```python
from build123d import *

# Parameters (mm, degrees)
SKETCH_1_W          = 83
SKETCH_1_H          = 28
EXTRUDE_1_DEPTH     = 5
SKETCH_2_R          = 2
CUT_EXTRUDE_1_DEPTH = 45.082309377
EXTRUDE_2_DEPTH     = 5
CUT_EXTRUDE_3_DEPTH = 156.991954214
FILLET_4_R          = 30
FILLET_5_R          = 20
SKETCH_6_R          = 2
CUT_EXTRUDE_4_DEPTH = 156.991954214
EXTRUDE_3_DEPTH     = 5
FILLET_7_R          = 10
SKETCH_8_R          = 5
CUT_EXTRUDE_5_DEPTH = 149.879193137
FILLET_8_R          = 20


with BuildPart() as part:
    # 草图1 → 凸台-拉伸1 (new body)
    with BuildSketch(Plane.XY):
        Rectangle(SKETCH_1_W, SKETCH_1_H)
    extrude(amount=EXTRUDE_1_DEPTH)

    # 草图2 → 切除-拉伸1 (cut, through all)
    with BuildSketch(Plane.XY.offset(5)):
        with Locations((6.5, 8)):
            Circle(SKETCH_2_R)
        with Locations((31.5, 8)):
            Circle(SKETCH_2_R)
        with Locations((31.5, -8)):
            Circle(SKETCH_2_R)
        with Locations((6.5, -8)):
            Circle(SKETCH_2_R)
    extrude(amount=-CUT_EXTRUDE_1_DEPTH, mode=Mode.SUBTRACT)

    # 草图3 → 凸台-拉伸2 (add)
    with BuildSketch(Plane(origin=(0, 0, 0), x_dir=(-1, 0, 0), z_dir=(0, 0, -1))):
        Polygon((41.5, 14), (59.770308511, 144), (29.5, 94), (-41.5, 14), align=None)
    extrude(amount=-EXTRUDE_2_DEPTH)

    # 草图5 → 切除-拉伸3 (cut, through all)
    with BuildSketch(Plane.XY.offset(5)):
        Polygon((36.5, 26), (-11.5, 26), (-35.602469952, 115.951642448), align=None)
    extrude(amount=-CUT_EXTRUDE_3_DEPTH, mode=Mode.SUBTRACT)

    # 圆角4
    fillet_4_edges = [part.edges().sort_by_distance(p)[0] for p in [
        (30.85, 26, 2.5),
    ]]
    fillet(fillet_4_edges, radius=FILLET_4_R)

    # 圆角5
    fillet_5_edges = [part.edges().sort_by_distance(p)[0] for p in [
        (-11.5, 26, 2.5),
    ]]
    fillet(fillet_5_edges, radius=FILLET_5_R)

    # 草图6 → 切除-拉伸4 (cut, through all)
    with BuildSketch(Plane.XY.offset(5)):
        with Locations((-36.5, -8.5)):
            Circle(SKETCH_6_R)
        with Locations((-4.5, -8.5)):
            Circle(SKETCH_6_R)
        with Locations((-4.5, 6.5)):
            Circle(SKETCH_6_R)
        with Locations((-36.5, 6.5)):
            Circle(SKETCH_6_R)
    extrude(amount=-CUT_EXTRUDE_4_DEPTH, mode=Mode.SUBTRACT)

    # 草图7 → 凸台-拉伸3 (add)
    with BuildSketch(Plane.XY.offset(5)):
        with BuildLine():
            Line((-41.5, 14), (-41.5, -14))
            ThreePointArc((-41.5, -14), (-70.837432371, 62.663912318), (-59.770308511, 144))
            Line((-59.770308511, 144), (-41.5, 14))
        make_face()
    extrude(amount=-EXTRUDE_3_DEPTH)

    # 圆角7
    fillet_7_edges = [part.edges().sort_by_distance(p)[0] for p in [
        (-59.770308511, 144, 2.5),
    ]]
    fillet(fillet_7_edges, radius=FILLET_7_R)

    # 草图8 → 切除-拉伸5 (cut, through all)
    with BuildSketch(Plane.XY.offset(5)):
        with Locations((-59.455425686, 101)):
            Circle(SKETCH_8_R)
    extrude(amount=-CUT_EXTRUDE_5_DEPTH, mode=Mode.SUBTRACT)

    # 圆角8
    fillet_8_edges = [part.edges().sort_by_distance(p)[0] for p in [
        (41.5, 14, 2.5),
    ]]
    fillet(fillet_8_edges, radius=FILLET_8_R)


solid = part.part
```
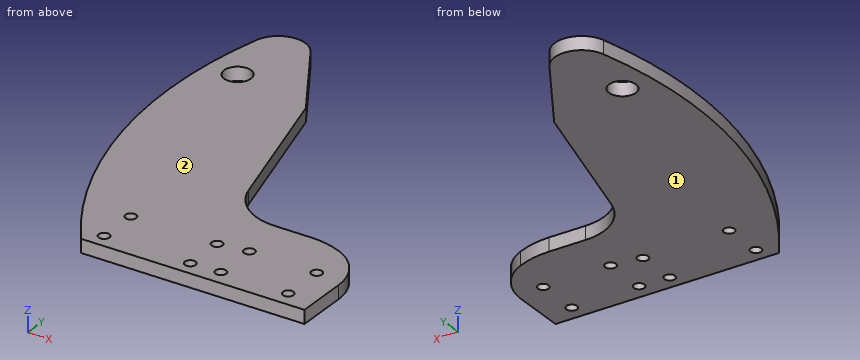
Check sheet for the modelled part. Datum: model origin and axes. Units: mm. Face numbers are marked on the shaded views. Coordinates: 2 decimals unless noted, no trailing zeros. Order: outer loops, then holes, each group sorted by start corner. A loop starts at its lowest first (then second) coordinate and runs counter-clockwise, first axis right, second up. Notation, with made-up numbers: M 44,71.5 L 65,71.5 A32 ccw 65,104.5 Z; hole C 53.25,53 d10. An arc over 180 degrees is marked long. One line per question, with ' | ' between items. Start each with the question number.
Item 1: Material ranges on line 1 (Y direction, x = 31.5, z = 3.05); line 2 (Y direction, x = 14.5, z = 3.05); line 3 (X direction, y = 79, z = 3.65), recorded low to high.
Item 2: Sectioned sample at D-D on z = 4. Count the separate pieces of the cut face and the enclosed holes in it, and give its area (3 significant figures).
Item 3: Sectioned sample at C-C on x = -58.5. Record the cut outline in (y, z), and give its area (3 significant figures).
Item 4: Sectioned sample at B-B on y = 101. Record the cut outline in (x, z), and give its area (3 significant figures).
Item 5: Mould release check, pull along Z, two halves, no side actions. Record for the marked faces 1 and 2: pulls with the +Z half, pulls with the -Z half, needs draft (parallel to the pull), parting line crosses it, or undercut.
Item 6: Gauge pin test, flat ends, axial feed: P1, Ø2.5, axis at x = 10, z = 2.5, coming from the +Y side; P2, Ø1.5, axis at y = 62, z = 1, coming from the +X side. Record the tip position at first contact, or that the pin passes through.
Item 7: Sectioned sample at A-A on x = -4.5. Record the cut outline in (y, z).
Answer below:
1) line 1: y = -14 to -10, -6 to 6, 10 to 22.43 | line 2: y = -14 to 26 | line 3: x = -71.91 to -25.7
2) separate pieces: 1 | enclosed holes: 9 | area: 7,870 mm^2
3) outline: M 16.34,0 L 96.09,0 L 96.09,5 L 16.34,5 Z; M 105.91,0 L 130.15,0 L 130.15,5 L 105.91,5 Z | area: 520 mm^2
4) outline: M -70.81,0 L -64.46,0 L -64.46,5 L -70.81,5 Z; M -54.46,0 L -33.74,0 L -33.74,5 L -54.46,5 Z | area: 135 mm^2
5) face 1: pulls with the -Z half | face 2: pulls with the +Z half
6) P1: stops at y = 26 | P2: stops at x = -20.95
7) outline: M -14,0 L -10.5,0 L -10.5,5 L -14,5 Z; M -6.5,0 L 4.5,0 L 4.5,5 L -6.5,5 Z; M 8.5,0 L 27.82,0 L 27.82,5 L 8.5,5 Z
